The model under review builds one solid part; all positions refer to its coordinate system, in mm. Face numbers are marked on the shaded views. A direction names the side the tool comes from. Round coordinates to 2 decimals unless told otherwise and drop trailing zeros. Write each loop counter-clockwise with the first axis right and the second up, starting at its lowest first coordinate (ties: lowest second). Pieces come first, ordered by that corner, then holes. Notation, with made-up numbers: (59, -31.5) -> (92, -31.5) arc R19 ccw to (92, -5.5) -> close; hole circle Ø8 at (-5.5, 5). An arc over 180 degrees is marked (long way). Answer as a JSON object with one key per item and string values. Group by question number.
1) To check wall thickness, follow probe 1 along X at (y, z) = (8, 6.25); probe 2 along Y at (x, z) = (8, 6.25); probe 3 along Y at (x, z) = (65, 4.5). State the ranges of each line that lie inside material, in increasing order. Write a range as [from, to].
2) Machinability: for the marked faces 1, 2 and 3, which of the approach directions +Z, -Z, +X, -X, +Y, -Y give a long, thin tool a straight path to every point of the face, cutting with its end or side? Answer none if there is none.
3) We need section A-A, the plane z = 4. Count the separate pieces of the cut face and the enclosed holes in it, then the cut area to 3 significant figures.
4) We need section C-C, the plane x = 73. Write out the cut boundary in (y, z), then the cut area to 3 significant figures.
5) We need section D-D, the plane y = 27.5. Write out the cut boundary in (x, z).
6) We need section B-B, the plane y = 50.5. Write out the cut boundary in (x, z).
7) Insertion check: pin 1 Ø1 at (x, z) = (47.5, -2.5) entering from -Y; pin 2 Ø8.5 at (x, y) = (23, 1.5) entering from +Z; pin 3 Ø1.6 at (x, y) = (-1, 28.5) entering from +Z. Each pin has a flat end and moves straight along its axis. Give the tip position at first contact, or say it passes through.
8) Mouldability with a two-part tool opening along X and no side actions: class the marked faces 4, 5, 6 and 7 as pulls with the +X half, pulls with the -X half, needs draft (parallel to the pull), parting line crosses it, or undercut.
from build123d import *

# Parameters (mm, degrees)
F2_DEPTH      = 3.5
F2_DEPTH_BACK = 10
F3_DEPTH      = 5
F5_START      = 5
F5_DEPTH      = 5
F7_DEPTH      = 10
F7_DEPTH_BACK = 3.5
F8_R          = 4
F10_DEPTH     = 94.501


with BuildPart() as f2:
    # F1 (on Top) → F2 (new body, two sides)
    with BuildSketch(Plane.XY) as f2_sk:
        with BuildLine():
            ThreePointArc((-3.25, -5.75), (-2.0784271247, -8.5784271247), (0.75, -9.75))
            Line((0.75, -9.75), (87.25, -9.75))
            ThreePointArc((87.25, -9.75), (90.0784271247, -8.5784271247), (91.25, -5.75))
            Line((91.25, -5.75), (91.25, 62.25))
            ThreePointArc((91.25, 62.25), (90.0784271247, 65.0784271247), (87.25, 66.25))
            Line((87.25, 66.25), (0.75, 66.25))
            ThreePointArc((0.75, 66.25), (-2.0784271247, 65.0784271247), (-3.25, 62.25))
            Line((-3.25, 62.25), (-3.25, -5.75))
        make_face()
    extrude(amount=-F2_DEPTH)
    extrude(f2_sk.sketch, amount=F2_DEPTH_BACK)

    # F0 (on Top) → F3 (cut)
    with BuildSketch(Plane.XY):
        with BuildLine():
            ThreePointArc((0, 4), (1.1715728753, 1.1715728753), (4, 0))
            Line((4, 0), (84, 0))
            ThreePointArc((84, 0), (86.8284271247, 1.1715728753), (88, 4))
            Line((88, 4), (88, 52.5))
            ThreePointArc((88, 52.5), (86.8284271247, 55.3284271247), (84, 56.5))
            Line((84, 56.5), (4, 56.5))
            ThreePointArc((4, 56.5), (1.1715728753, 55.3284271247), (0, 52.5))
            Line((0, 52.5), (0, 4))
        make_face()
    extrude(amount=F3_DEPTH, mode=Mode.SUBTRACT)

    # F4 (on Top) → F5 (cut)
    with BuildSketch(Plane.XY.offset(F5_START)):
        with BuildLine():
            ThreePointArc((0, -2.5), (1.1715728753, -5.3284271247), (4, -6.5))
            Line((4, -6.5), (84, -6.5))
            ThreePointArc((84, -6.5), (86.8284271247, -5.3284271247), (88, -2.5))
            Line((88, -2.5), (88, 59))
            ThreePointArc((88, 59), (86.8284271247, 61.8284271247), (84, 63))
            Line((84, 63), (4, 63))
            ThreePointArc((4, 63), (1.1715728753, 61.8284271247), (0, 59))
            Line((0, 59), (0, -2.5))
        make_face()
    extrude(amount=F5_DEPTH, mode=Mode.SUBTRACT)

    # F6 (on Top) → F7 (cut, two sides)
    with BuildSketch(Plane.XY) as f7_sk:
        with BuildLine():
            Line((33.0040588687, 0.4603501153), (29, -9.75))
            Line((29, -9.75), (44, -9.75))
            Line((44, -9.75), (59, -9.75))
            Line((59, -9.75), (54.9959411313, 0.4603501153))
            ThreePointArc((54.9959411313, 0.4603501153), (53.5257785273, 2.3046482764), (51.2720483373, 3))
            Line((51.2720483373, 3), (44, 3))
            Line((44, 3), (36.7279516627, 3))
            ThreePointArc((36.7279516627, 3), (34.4742214727, 2.3046482764), (33.0040588687, 0.4603501153))
        make_face()
    extrude(amount=F7_DEPTH, mode=Mode.SUBTRACT)
    extrude(f7_sk.sketch, amount=-F7_DEPTH_BACK, mode=Mode.SUBTRACT)

    # F8
    f8_edges = [f2.edges().sort_by_distance(p)[0] for p in [
        (59, -9.75, 3.25),
        (29, -9.75, 3.25),
    ]]
    fillet(f8_edges, radius=F8_R)

    # F9 (on face) → F10 (cut, through all)
    with BuildSketch(Plane(origin=(-3.25, 0, 0), x_dir=(0, -1, 0), z_dir=(-1, 0, 0))):
        Polygon((-20.75, 2.5), (-18.25, 10), (-28.25, 10), (-38.25, 10), (-35.75, 2.5), (-28.25, 2.5), align=None)
    extrude(amount=-F10_DEPTH, mode=Mode.SUBTRACT)


solid = f2.part
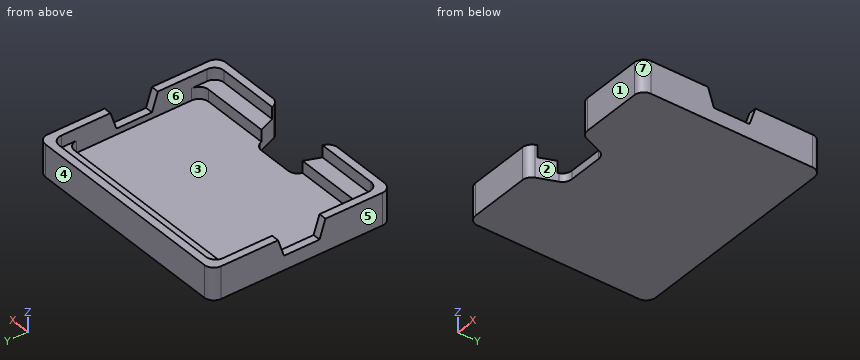
Here are the results:
{
 "1": {"probe 1": "x = [-3.25, 0], [88, 91.25]", "probe 2": "y = [-9.75, -6.5], [63, 66.25]", "probe 3": "y = [-9.75, 0], [56.5, 66.25]"},
 "2": {"face 1": "+Z, -Z, +X, -X, -Y", "face 2": "+Z, -Z, -Y", "face 3": "+Z"},
 "3": {"separate pieces": "3", "enclosed holes": "0", "area": "1,850 mm^2"},
 "4": {"outline": "(-9.75, -3.5) -> (66.25, -3.5) -> (66.25, 10) -> (63, 10) -> (63, 5) -> (56.5, 5) -> (56.5, 0) -> (0, 0) -> (0, 5) -> (-6.5, 5) -> (-6.5, 10) -> (-9.75, 10) -> close", "area": "396 mm^2"},
 "5": {"outline": "(-3.25, -3.5) -> (91.25, -3.5) -> (91.25, 2.5) -> (88, 2.5) -> (88, 0) -> (0, 0) -> (0, 2.5) -> (-3.25, 2.5) -> close"},
 "6": {"outline": "(-3.25, -3.5) -> (91.25, -3.5) -> (91.25, 10) -> (88, 10) -> (88, 0) -> (0, 0) -> (0, 10) -> (-3.25, 10) -> close"},
 "7": {"pin 1": "stops at y = 3", "pin 2": "stops at z = 5", "pin 3": "stops at z = 2.5"},
 "8": {"face 4": "needs draft", "face 5": "pulls with the -X half", "face 6": "undercut", "face 7": "pulls with the +X half"}
}
